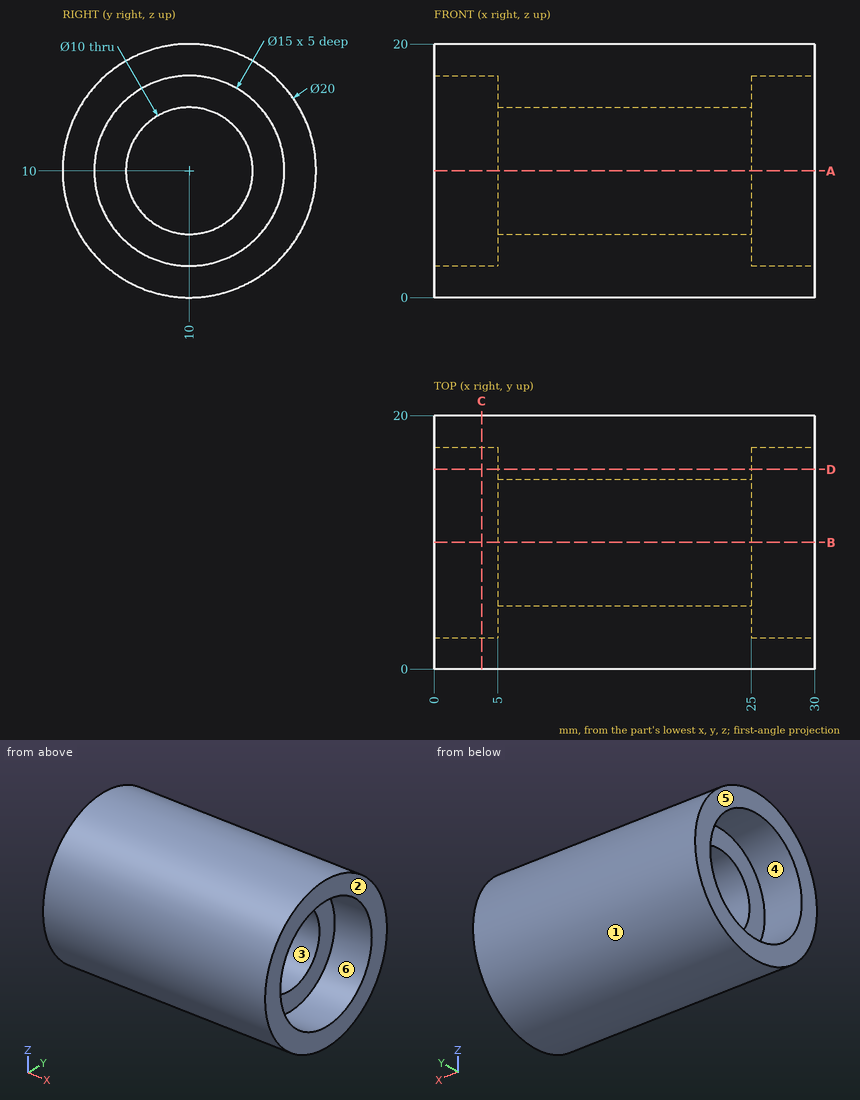
Could you check a few things on this drawing? It's one solid part, dimensions in mm from its lowest x, y, z. A direction names the side the tool comes from. Give positions to 0.01 mm unless a question says otherwise; leave off trailing zeros. Order: outer loops, then holes, each group sorted by start corner. A loop starts at its lowest first (then second) coordinate and runs counter-clockwise, first axis right, second up. Notation, with made-up numbers: M 71.25,37.5 L 92.25,37.5 A22 cw 92.25,51.5 Z; hole C 0.25,59.5 d3. An arc over 180 degrees is marked long. Use one line per item in the form item = value.
Item 1: Thinking about a two-plate mould opening in Y: for the marked faces 1, 2 and 3, which applies, pulls with the +Y half, pulls with the -Y half, needs draft (parallel to the pull), parting line crosses it, or undercut?
Values follow:
face_1 = parting line crosses it
face_2 = needs draft
face_3 = undercut
Item 2: If I drill on line 1 along Z through (x, y) = (28.6, 10); line 2 along Z through (x, y) = (10.75, 10); line 3 along X through (y, z) = (15.5, 13.5), over which ranges is the centre line in solid material (lowest first)? Write a range as [from, to].
Values follow:
line_1 = [0, 2.5], [17.5, 20]
line_2 = [0, 5], [15, 20]
line_3 = [5, 25]
Item 3: Will these pins go through, and if not, where does the flat tip stop? pin 1 Ø10 at (x, z) = (11, 12.5) entering from -Y; pin 2 Ø5 at (x, z) = (6.5, 3.5) entering from -Y; pin 3 Ø5 at (y, z) = (7, 10) entering from +X; pin 4 Ø2 at (x, y) = (7, 13) entering from +Z.
Values follow:
pin_1 = 0
pin_2 = 0.83
pin_3 = 25
pin_4 = 19.8
Item 4: For the marked faces 4, 5 and 6, which set-ups out of +Z, -Z, +X, -X, +Y, -Y let a thin tool reach every point of the face, with its end or its side?
Values follow:
face_4 = -X
face_5 = +Z, -Z, -X, +Y, -Y
face_6 = +X
Item 5: If we section it at A-A, the plane z = 10: Write out the boundary of the cut face in (x, y), and give its area (3 significant figures).
Values follow:
outline = M 0,0 L 30,0 L 30,2.5 L 25,2.5 L 25,5 L 5,5 L 5,2.5 L 0,2.5 Z; M 0,17.5 L 5,17.5 L 5,15 L 25,15 L 25,17.5 L 30,17.5 L 30,20 L 0,20 Z
area = 250 mm^2
Item 6: If we section it at C-C, the plane x = 3.75: Write out the boundary of the cut face in (y, z), and give its area (3 significant figures).
Values follow:
outline = C 10,10 d20; hole C 10,10 d15
area = 137 mm^2
Item 7: If we section it at D-D, the plane y = 15.75: Write out the boundary of the cut face in (x, z), and give its area (3 significant figures).
Values follow:
outline = M 0,1.82 L 30,1.82 L 30,5.18 L 25,5.18 L 25,14.82 L 30,14.82 L 30,18.18 L 0,18.18 L 0,14.82 L 5,14.82 L 5,5.18 L 0,5.18 Z
area = 395 mm^2
